Read the model definition and answer for the solid it produces. Units are mm, in the model's axes. Face numbers are marked on the shaded views. Give positions to 0.01 mm unless a question says otherwise; leave off trailing zeros. Loops run counter-clockwise (first coordinate to the right, second up) from the corner with the lowest first, then second, coordinate; pieces in that order, holes last. Notation, with made-up numbers: (48, -12) -> (65, -12) arc R26 cw to (65, 2) -> close; hole circle Ø6 at (77.5, 71.25). An arc over 180 degrees is marked (long way). Return JSON: item names as keys, results as strings. Group by question number.
from build123d import *

# Parameters (mm, degrees)
F0_W       = 100
F0_H       = 100
F1_DEPTH   = 50
F5_D       = 80
F5_ON_F4_D = 80
F5_ON_F3_D = 80


with BuildPart() as f1:
    # F0 (on Front) → F1 (new body, symmetric)
    with BuildSketch(Plane.XZ):
        Rectangle(F0_W, F0_H)
    extrude(amount=F1_DEPTH, both=True)

    # F5 (through all)
    with Locations(Plane.XZ.offset(50)):
        with Locations((0, 0)):
            Hole(F5_D / 2)

    # F5 on F4 (through all)
    with Locations(Plane.XY.offset(50)):
        with Locations((0, 0)):
            Hole(F5_ON_F4_D / 2)

    # F5 on F3 (through all)
    with Locations(Plane.YZ.offset(50)):
        with Locations((0, 0)):
            Hole(F5_ON_F3_D / 2)


solid = f1.part
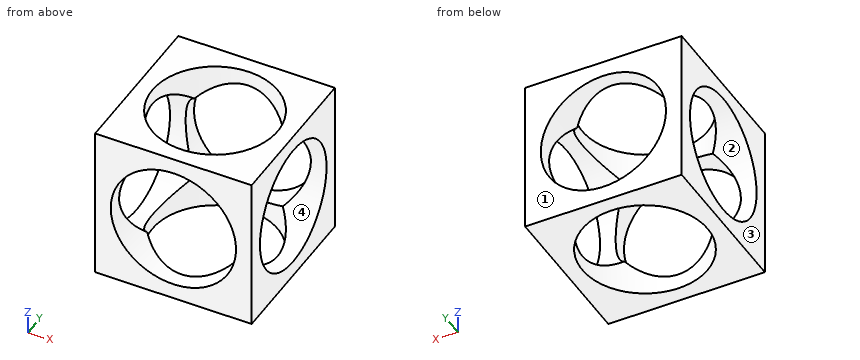
1. Section C-C on y = 42 is taken. Determine the outline of the cut face in (x, z), then the cut area to 3 significant figures.
2. Section A-A on y = 0 is taken. Determine the outline of the cut face in (x, z).
3. Section D-D on x = -37 is taken. Determine the outline of the cut face in (y, z).
4. Straight lines are drawn through the part: line 1 (Y direction, x = -41, z = 0); line 2 (Z direction, x = -25, y = -36). For each, find the intervals that lie inside material, in ascending order. Write a range as from..to.
5. Determine the mould class of the marked faces 1, 2, 3 and 4 for opening direction Y: pulls with the +Y half, pulls with the -Y half, needs draft (parallel to the pull), parting line crosses it, or undercut.
6. Section B-B on x = -17 is taken. Determine the outline of the cut face in (y, z), then the cut area to 3 significant figures.
Completed:
{
 "1": {"outline": "(-50, -50) -> (50, -50) -> (50, 50) -> (-50, 50) -> close; hole circle Ø80 at (0, 0)", "area": "4,970 mm²"},
 "2": {"outline": "(-50, -50) -> (-40, -50) -> (-40, -40) -> (-50, -40) -> close; (-50, 40) -> (-40, 40) -> (-40, 50) -> (-50, 50) -> close; (40, -50) -> (50, -50) -> (50, -40) -> (40, -40) -> close; (40, 40) -> (50, 40) -> (50, 50) -> (40, 50) -> close"},
 "3": {"outline": "(-50, -50) -> (-15.2, -50) -> (-15.2, -37) arc R40 cw to (-37, -15.2) -> (-50, -15.2) -> close; (-50, 15.2) -> (-37, 15.2) arc R40 cw to (-15.2, 37) -> (-15.2, 50) -> (-50, 50) -> close; (15.2, -50) -> (50, -50) -> (50, -15.2) -> (37, -15.2) arc R40 cw to (15.2, -37) -> close; (15.2, 37) arc R40 cw to (37, 15.2) -> (50, 15.2) -> (50, 50) -> (15.2, 50) -> close"},
 "4": {"line 1": "y = -50..-40, 40..50", "line 2": "z = -50..-31.22, 31.22..50"},
 "5": {"face 1": "pulls with the +Y half", "face 2": "undercut", "face 3": "needs draft", "face 4": "undercut"},
 "6": {"outline": "(-50, -50) -> (-36.21, -50) -> (-36.21, -36.21) -> (-50, -36.21) -> close; (-50, 36.21) -> (-36.21, 36.21) -> (-36.21, 50) -> (-50, 50) -> close; (36.21, -50) -> (50, -50) -> (50, -36.21) -> (36.21, -36.21) -> close; (36.21, 36.21) -> (50, 36.21) -> (50, 50) -> (36.21, 50) -> close", "area": "761 mm²"}
}
